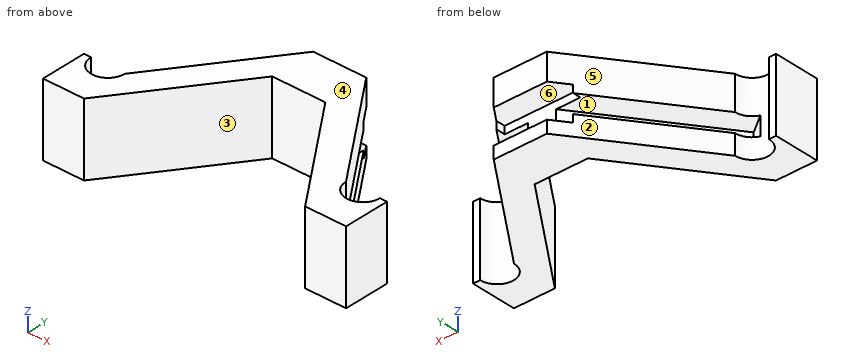
from build123d import *

# Parameters (mm, degrees)
BOSS_EXTRUDE1_DEPTH = 30
SKETCH3_W           = 31.24049206
SKETCH3_H           = 13.927985749
CUT_EXTRUDE1_DEPTH  = 10
SKETCH4_W           = 7.689934576
SKETCH4_H           = 62.184409798
CUT_EXTRUDE2_DEPTH  = 10


with BuildPart() as part:
    # Sketch2 → Boss-Extrude1 (new body)
    with BuildSketch(Plane.XY):
        with BuildLine():
            Line((-10.970149254, 0), (0, 0))
            Line((0, 0), (0, 18.805970149))
            Line((0, 18.805970149), (-10.970149254, 18.805970149))
            Line((-10.970149254, 18.805970149), (-45.656716418, -29.149253731))
            ThreePointArc((-45.656716418, -29.149253731), (-52.656716418, -36.149253731), (-59.656716418, -29.149253731))
            Line((-59.656716418, -29.149253731), (-62.582089552, -29.149253731))
            Line((-62.582089552, -29.149253731), (-62.582089552, -47.955223881))
            Line((-62.582089552, -47.955223881), (-45.656716418, -47.955223881))
            Line((-45.656716418, -47.955223881), (-10.970149254, 0))
        make_face()
        with BuildLine():
            Line((0, 0), (10.970149254, 0))
            Line((10.970149254, 0), (45.656716418, -47.955223881))
            Line((45.656716418, -47.955223881), (62.582089552, -47.955223881))
            Line((62.582089552, -47.955223881), (62.582089552, -29.149253731))
            Line((62.582089552, -29.149253731), (59.656716418, -29.149253731))
            ThreePointArc((59.656716418, -29.149253731), (52.656716418, -36.149253731), (45.656716418, -29.149253731))
            Line((45.656716418, -29.149253731), (10.970149254, 18.805970149))
            Line((10.970149254, 18.805970149), (0, 18.805970149))
            Line((0, 18.805970149), (0, 0))
        make_face()
    extrude(amount=BOSS_EXTRUDE1_DEPTH)

    # Sketch3 → Cut-Extrude1 (cut)
    with BuildSketch(Plane(origin=(0, 18.805970149, 0), x_dir=(1, 0, 0), z_dir=(0, 1, 0))):
        with Locations((-0.199336915, -12.101360071)):
            Rectangle(SKETCH3_W, SKETCH3_H)
    extrude(amount=-CUT_EXTRUDE1_DEPTH, mode=Mode.SUBTRACT)

    # Sketch4 → Cut-Extrude2 (cut)
    with BuildSketch(Plane(origin=(-16.132519574, 11.668837688, 0), x_dir=(0, 0, 1), z_dir=(-0.8102600819579188, 0.5860704732244638, 0))):
        with Locations((12.122562235, -27.26241609)):
            Rectangle(SKETCH4_W, SKETCH4_H)
    cut_extrude2 = extrude(amount=-CUT_EXTRUDE2_DEPTH, mode=Mode.SUBTRACT)

    # Mirror1: Cut-Extrude2 across plane
    add(cut_extrude2.mirror(Plane(origin=(0, 0, 0), x_dir=(0, 0, 1), z_dir=(1, 0, 0))), mode=Mode.SUBTRACT)


solid = part.part
For this review, take the finished solid that the model builds, in its own axes (mm). Face numbers are marked on the shaded views. A direction names the side the tool comes from. Round coordinates to 2 decimals unless told otherwise and drop trailing zeros. Write each loop counter-clockwise with the first axis right and the second up, starting at its lowest first coordinate (ties: lowest second). Pieces come first, ordered by that corner, then holes. Notation, with made-up numbers: (-17.75, 62) - (17.25, 62) arc R15 cw to (17.25, 77) - close; hole circle Ø2 at (54.5, 31). An arc over 180 degrees is marked (long way). Write item = value, one per line. Start each with the question number.
1. For pin 1 Ø1.5 at (y, z) = (11.5, 18) entering from -X; pin 2 Ø1.5 at (x, z) = (-60.5, 20) entering from +Y; pin 3 Ø2.5 at (y, z) = (9.5, 7) entering from +X, all flat-tipped, find the tip position at first contact; note any pin that passes through.
2. Consider section B-B on z = 27.75. State the section outline as (x, y) points, plus the area to 3 significant figures.
3. Draft analysis for pull direction Z (two halves, no side actions). For the marked faces 4, 5 and 6, state which applies: released by +Z, released by -Z, zero draft, split by the parting line, or undercut.
4. Consider section D-D on x = 1. State the section outline as (y, z) points.
5. Consider section C-C on y = 14.5. State the section outline as (x, z) points.
6. For the marked faces 1, 2 and 3, list the 3-axis set-ups (+Z, -Z, +X, -X, +Y, -Y) from which the entire face can be reached by the end or side of a thin tool; tool diameter is ignored.
7. Wall thickness on L1, parallel to X at y = -32, z = 16.25; L2, parallel to Z at x = -14, y = 4; L3, parallel to X at y = -24.5, z = 23.5: over which ranges is each line inside the solid? List them lowest first.
8. Consider section A-A on y = -38.5. State the section outline as (x, z) points, plus the area to 3 significant figures.
Evaluation:
q1.pin_1 = -16.8
q1.pin_2 = -29.15
q1.pin_3 = 18.61
q2.outline = (-62.58, -47.96) - (-45.66, -47.96) - (-10.97, 0) - (10.97, 0) - (45.66, -47.96) - (62.58, -47.96) - (62.58, -29.15) - (59.66, -29.15) arc R7 cw to (45.66, -29.15) - (10.97, 18.81) - (-10.97, 18.81) - (-45.66, -29.15) arc R7 cw to (-59.66, -29.15) - (-62.58, -29.15) - close
q2.area = 2,200 mm2
q3.face_4 = released by +Z
q3.face_5 = zero draft
q3.face_6 = undercut
q4.outline = (0, 0) - (18.81, 0) - (18.81, 5.14) - (8.81, 5.14) - (8.81, 19.07) - (18.81, 19.07) - (18.81, 30) - (0, 30) - close
q5.outline = (-14.08, 0) - (14.08, 0) - (14.08, 5.14) - (-14.08, 5.14) - close; (-14.08, 19.07) - (14.08, 19.07) - (14.08, 30) - (-14.08, 30) - close
q6.face_1 = +Y
q6.face_2 = +Z, -Z, -X, +Y
q6.face_3 = +Z, -Z, -Y
q7.L1 = -62.58 to -59.05, -46.26 to -34.12, 34.12 to 46.26, 59.05 to 62.58
q7.L2 = 0 to 8.28, 15.97 to 30
q7.L3 = -42.29 to -28.69, 28.69 to 42.29
q8.outline = (-62.58, 0) - (-38.82, 0) - (-38.82, 30) - (-62.58, 30) - close; (38.82, 0) - (62.58, 0) - (62.58, 30) - (38.82, 30) - close; hole (-46.34, 8.28) - (-40.08, 8.28) - (-40.08, 15.97) - (-46.34, 15.97) - close; hole (40.08, 8.28) - (46.34, 8.28) - (46.34, 15.97) - (40.08, 15.97) - close
q8.area = 1,330 mm2
